The figure shows three views and two pictorial views of one solid part (mm, origin at its lowest corner). Answer the questions. Coordinates: 2 decimals unless noted, no trailing zeros. Write each loop counter-clockwise with the first axis right and the second up, starting at its lowest first coordinate (ties: lowest second). Pieces come first, ordered by that corner, then holes. Notation, with made-up numbers: (-16.75, 33.25) - (12.25, 33.25) arc R30 ccw to (12.25, 59.25) - close; hole circle Ø4 at (34, 7.25). An arc over 180 degrees is marked (long way). Use a Markdown table: item, result. Add a question column.
(1) Given pin 1 Ø6 at (x, y) = (181.5, 44.5) entering from +Z, flat-ended and moving along its own axis, determine where the tip first touches the part or whether it passes through.
(2) Find the intervals of material crossed by line 1 (Y direction, x = 191.77, z = 0.65); line 2 (X direction, y = 49, z = 1.8); line 3 (Y direction, x = 75.5, z = 1) (1 decimal), in increasing order. Write a range as from..to.
(3) The part is cut by section C-C, the plane y = 107. Give the vertices of the cut face in (x, z), then the cut area to 3 significant figures.
(4) The part is cut by section D-D, the plane x = 195. Give the vertices of the cut face in (y, z).
(5) The part is cut by section A-A, the plane x = 166.37. Give the vertices of the cut face in (y, z), then the cut area to 3 significant figures.
(6) The part is cut by section B-B, the plane z = 0.5. State how many separate pieces and enclosed holes the cut face has, then the cut area to 3 significant figures.
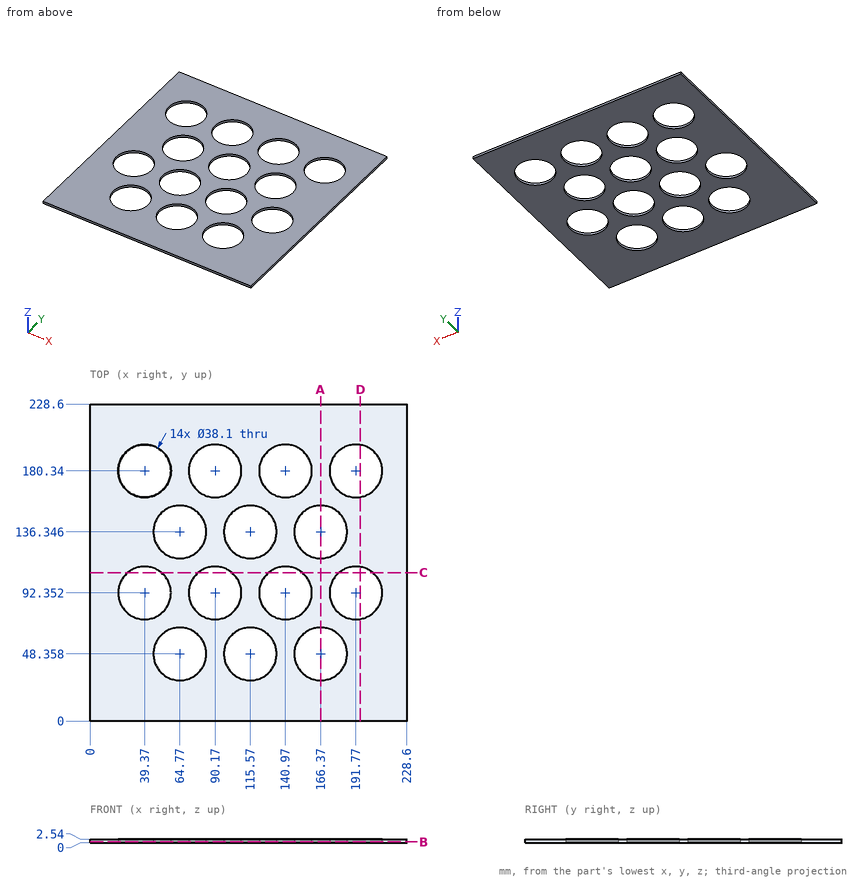
Model answer:
| question | item | result |
|---|---|---|
| 1 | pin 1 | through |
| 2 | line 1 | 0..73.3, 111.4..161.29, 199.39..228.6 |
| 2 | line 2 | 0..45.73, 83.81..96.53, 134.61..147.33, 185.41..228.6 |
| 2 | line 3 | 0..32.6, 64.1..80.2, 104.5..120.6, 152.1..168.2, 192.5..228.6 |
| 3 | outline | (0, 0) - (27.19, 0) - (27.19, 2.54) - (0, 2.54) - close; (51.55, 0) - (77.99, 0) - (77.99, 2.54) - (51.55, 2.54) - close; (102.35, 0) - (128.79, 0) - (128.79, 2.54) - (102.35, 2.54) - close; (153.15, 0) - (179.59, 0) - (179.59, 2.54) - (153.15, 2.54) - close; (203.95, 0) - (228.6, 0) - (228.6, 2.54) - (203.95, 2.54) - close |
| 3 | area | 333 mm^2 |
| 4 | outline | (0, 0) - (73.58, 0) - (73.58, 2.54) - (0, 2.54) - close; (111.13, 0) - (161.57, 0) - (161.57, 2.54) - (111.13, 2.54) - close; (199.11, 0) - (228.6, 0) - (228.6, 2.54) - (199.11, 2.54) - close |
| 5 | outline | (0, 0) - (29.31, 0) - (29.31, 2.54) - (0, 2.54) - close; (67.41, 0) - (117.3, 0) - (117.3, 2.54) - (67.41, 2.54) - close; (155.4, 0) - (228.6, 0) - (228.6, 2.54) - (155.4, 2.54) - close |
| 5 | area | 387 mm^2 |
| 6 | separate pieces | 1 |
| 6 | enclosed holes | 14 |
| 6 | area | 36,300 mm^2 |
